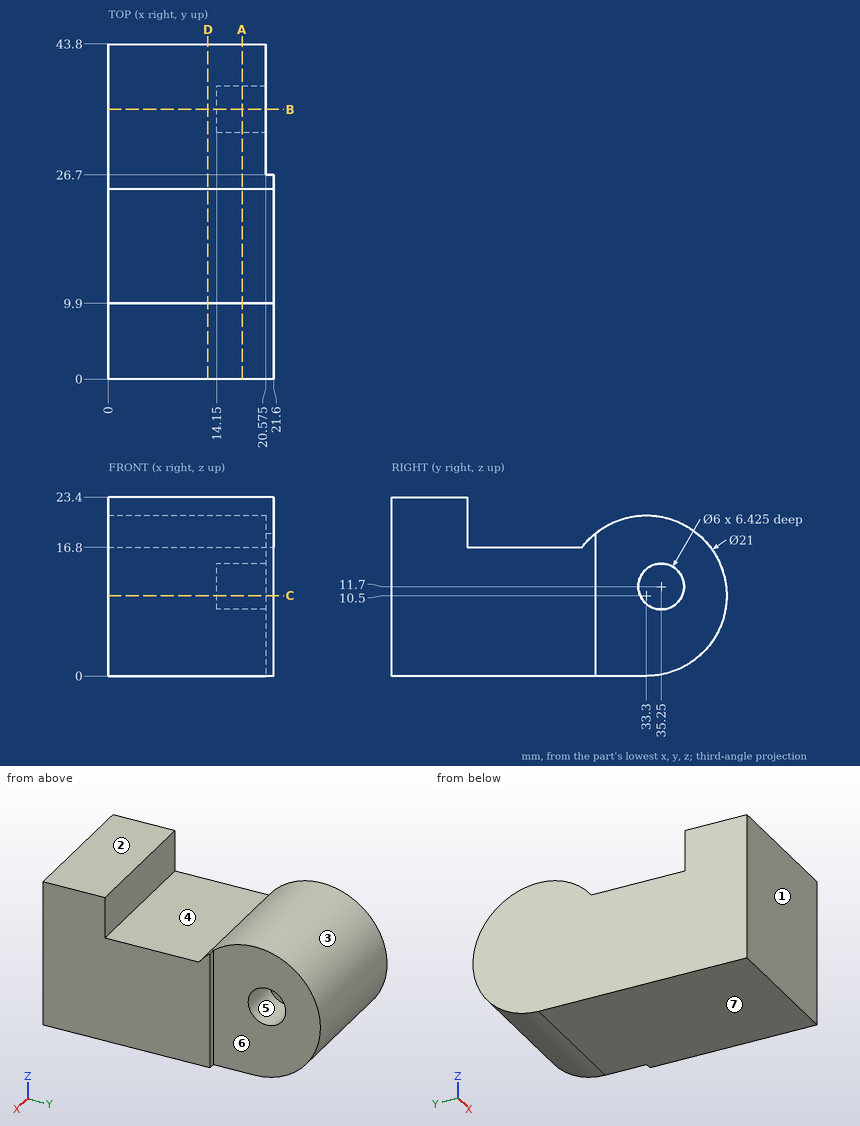
The figure shows three views and two pictorial views of one solid part (mm, origin at its lowest corner). Answer the questions. A direction names the side the tool comes from. Round coordinates to 2 decimals unless told otherwise and drop trailing zeros. Write each loop counter-clockwise with the first axis right and the second up, starting at its lowest first coordinate (ties: lowest second). Pieces come first, ordered by that corner, then holes. Notation, with made-up numbers: (87, 63.25) - (121, 63.25) arc R23 cw to (121, 99.25) - close; hole circle Ø1 at (40.5, 62.5). An arc over 180 degrees is marked (long way). Use one line per item in the form item = value. Start each with the question number.
Item 1: Flat-ended cylindrical pins translate along their axes: pin 1 Ø3 at (y, z) = (35, 10.5) entering from +X; pin 2 Ø3.5 at (x, z) = (7.5, 19.5) entering from +Y; pin 3 Ø12 at (x, y) = (2.5, 20) entering from +Z. Find the tip coordinate at first contact, or state that the pin passes through.
Item 2: Find the intervals of material crossed by line 1 (X direction, y = 29, z = 6.25) (3 decimals); line 2 (Z direction, x = 12.25, y = 15); line 3 (Y direction, x = 16, z = 11.7), in increasing order. Write a range as [from, to].
Item 3: Determine the mould class of the marked faces 1, 2 and 3 for opening direction Y: +Y half, -Y half, draft (parallel to the pull), parting line (faces both ways), or undercut.
Item 4: A cutting plane is placed at D-D (x = 13). Write down the section's boundary in (y, z).
Item 5: A cutting plane is placed at B-B (y = 35.25). Write down the section's boundary in (x, z) (3 decimals), plus the area to 3 significant figures.
Item 6: A cutting plane is placed at C-C (z = 10.5). Write down the section's boundary in (x, y) (3 decimals), plus the area to 3 significant figures.
Item 7: A tool of negligible diameter and unlimited length cuts with its end or side. For the marked faces 4, 5, 6 and 7, from which of +Z, -Z, +X, -X, +Y, -Y can it reach the whole face along a straight path? Write none if from no direction.
Item 8: A cutting plane is placed at A-A (x = 17.5). Write down the section's boundary in (y, z), plus the area to 3 significant figures.
The answers:
q1.pin_1 = 14.15
q1.pin_2 = 40.9
q1.pin_3 = 18.05
q2.line_1 = [0, 20.575]
q2.line_2 = [0, 16.8]
q2.line_3 = [0, 32.25], [38.25, 43.73]
q3.face_1 = -Y half
q3.face_2 = draft
q3.face_3 = undercut
q4.outline = (0, 0) - (33.3, 0) arc R10.5 ccw (long way) to (24.9, 16.8) - (9.9, 16.8) - (9.9, 23.4) - (0, 23.4) - close
q5.outline = (0, 0.183) - (20.575, 0.183) - (20.575, 8.7) - (14.15, 8.7) - (14.15, 14.7) - (20.575, 14.7) - (20.575, 20.817) - (0, 20.817) - close
q5.area = 386 mm^2
q6.outline = (0, 0) - (21.6, 0) - (21.6, 26.7) - (20.575, 26.7) - (20.575, 32.5) - (14.15, 32.5) - (14.15, 38) - (20.575, 38) - (20.575, 43.8) - (0, 43.8) - close
q6.area = 893 mm^2
q7.face_4 = +Z, +X, -X
q7.face_5 = +X
q7.face_6 = +Z, -Z, +X, +Y
q7.face_7 = -Z, +X, -X, +Y, -Y
q8.outline = (0, 0) - (33.3, 0) arc R10.5 ccw (long way) to (24.9, 16.8) - (9.9, 16.8) - (9.9, 23.4) - (0, 23.4) - close; hole circle Ø6 at (35.25, 11.7)
q8.area = 794 mm^2
